Read the model definition and answer for the solid it produces. Units are mm, in the model's axes. A direction names the side the tool comes from. Round coordinates to 2 decimals unless told otherwise and drop trailing zeros. Loops run counter-clockwise (first coordinate to the right, second up) from the corner with the lowest first, then second, coordinate; pieces in that order, holes last. Notation, with made-up numbers: (9.25, 62.5) -> (55.25, 62.5) arc R23 ccw to (55.25, 98.5) -> close; hole circle Ø7 at (27, -6). An arc over 180 degrees is marked (long way). Put each result on its own line as item: value.
Solid Edge part; units mm, degrees
sketch "Sketch1" plane through (0, 0, 0) normal (0, -1, 0) x (1, 0, 0)
  line L0 (-45, 15) -> (-45, 45)
  line L1 (-45, 45) -> (0, 45)
  line L2 (0, 45) -> (0, 0)
  line L3 (-30, 0) -> (0, 0)
  arc A0 (-30, 0) -> (-45, 15) centre (-30, 15) cw
extrude "ExtrudedProtrusion_1" add sketch "Sketch1" along normal mid plane 30
hole "Hole_1" at (-7, 0, 45) direction (0, 0, -1) diameter 12 depth 15
hole "Hole_2" at (0, 0, 9.5) direction (-1, 0, 0) diameter 15 depth 12
hole "Hole_3" at (-7, 0, 30) direction (0, 0, -1) diameter 7 end up to next
fillet "Round_1" radius 15 1 edges at (0, 0, 45)
hole "Hole_4" at (-30, -15, 15) direction (0, 1, 0) diameter 15 end up to next
sketch "Sketch2" plane through (0, 0, 0) normal (0, -1, 0) x (1, 0, 0)
  circle A0 centre (-30, 15) radius 7.5
  circle A1 centre (-30, 15) radius 5
extrude "ExtrudedProtrusion_2" add sketch "Sketch2" along normal mid plane 5
Item 1: The part is cut by section C-C (y = 0). Determine the outline of the cut face in (x, z).
Derived:
outline: (-45, 15) arc R15 ccw to (-30, 0) -> (0, 0) -> (0, 2) -> (-12, 2) -> (-12, 17) -> (-10.5, 17) -> (-10.5, 30) -> (-13, 30) -> (-13, 44.87) arc R15 ccw to (-15, 45) -> (-45, 45) -> close; (-3.5, 17) -> (0, 17) -> (0, 30) arc R15 ccw to (-1, 35.39) -> (-1, 30) -> (-3.5, 30) -> close; hole circle Ø10 at (-30, 15)
Item 2: Flat-ended cylindrical pins translate along their axes: pin 1 Ø5 at (y, z) = (-8.5, 10.5) entering from -X; pin 2 Ø4.5 at (y, z) = (0.5, 12.5) entering from +X; pin 3 Ø4 at (x, y) = (-34, -1) entering from -Z. Find the tip coordinate at first contact, or state that the pin passes through.
Derived:
pin 1: stops at x = -44.87
pin 2: stops at x = -12
pin 3: stops at z = 0.13
Item 3: Which of the six approach directions +Z, -Z, +X, -X, +Y, -Y give full straight-line access (tool end or side, diameter ignored) to faces 4 (the cylindrical face through (-34.564, -8.838, 20.952)), 5 (the cylindrical face through (-34.564, 8.663, 20.952)), 6 (the cylindrical face through (-6.08, 2.87, 2.57)), 7 (the cylindrical face through (-10.417, 0.759, 23.164))?
Derived:
face 4: -Y
face 5: +Y
face 6: +X
face 7: +Z
Item 4: Find the intervals of material crossed by line 1 along X through (y, z) = (5.5, 15); line 2 along Z through (x, y) = (-3, 0); line 3 along Y through (x, z) = (-9.5, 9.5), in increasing order.
Derived:
line 1: x = -45 to -37.5, -22.5 to 0
line 2: z = 0 to 2, 17 to 30
line 3: y = -15 to -7.5, 7.5 to 15
Item 5: The part is cut by section A-A (y = 8.5). Determine the outline of the cut face in (x, z), then the cut area to 3 significant figures.
Derived:
outline: (-45, 15) arc R15 ccw to (-30, 0) -> (0, 0) -> (0, 30) arc R15 ccw to (-15, 45) -> (-45, 45) -> close; hole circle Ø15 at (-30, 15)
area: 1,750 mm^2
Item 6: For a pull along Z with two mould halves and no side action, classify faces 1 (the flat face through (-32, 2.5, 10)), 2 (the cylindrical face through (-40.49, 0.21, 4.28)), 3 (the flat face through (-22, 15, 22)) as pulls with the +Z half, pulls with the -Z half, needs draft (parallel to the pull), parting line crosses it, or undercut.
Derived:
face 1: undercut
face 2: pulls with the -Z half
face 3: needs draft
Item 7: The part is cut by section D-D (x = -9.5). Determine the outline of the cut face in (y, z), then the cut area to 3 significant figures.
Derived:
outline: (-15, 0) -> (15, 0) -> (15, 43.96) -> (5.45, 43.96) -> (5.45, 30) -> (2.45, 30) -> (2.45, 16.59) arc R7.5 cw (long way) to (-2.45, 16.59) -> (-2.45, 30) -> (-5.45, 30) -> (-5.45, 43.96) -> (-15, 43.96) -> close
area: 925 mm^2
Item 8: The part is cut by section B-B (z = 13). Determine the outline of the cut face in (x, y).
Derived:
outline: (-44.87, -15) -> (-37.23, -15) -> (-37.23, -2.5) -> (-34.58, -2.5) -> (-34.58, 2.5) -> (-37.23, 2.5) -> (-37.23, 15) -> (-44.87, 15) -> close; (-25.42, -2.5) -> (-22.77, -2.5) -> (-22.77, -15) -> (0, -15) -> (0, -6.63) -> (-12, -6.63) -> (-12, 6.63) -> (0, 6.63) -> (0, 15) -> (-22.77, 15) -> (-22.77, 2.5) -> (-25.42, 2.5) -> close
